```python
from build123d import *

# Parameters (mm, degrees)
SKETCH1_W           = 42
SKETCH1_H           = 22.5
BOSS_EXTRUDE1_DEPTH = 5.75
SKETCH2_W           = 10.5
SKETCH2_H           = 21.5
CUT_EXTRUDE1_DEPTH  = 4
SKETCH3_R           = 1
BOSS_EXTRUDE2_DEPTH = 8
SKETCH4_R           = 0.5
BOSS_EXTRUDE3_DEPTH = 8
SKETCH5_R           = 1.030633651
SKETCH5_W           = 20.392034512
SKETCH5_H           = 11.098868447
CUT_EXTRUDE2_DEPTH  = 0.5
SKETCH9_W           = 11.5
SKETCH9_H           = 22.5
SKETCH9_W_2         = 10.5
SKETCH9_H_2         = 21.5
CUT_EXTRUDE5_DEPTH  = 3.5
SKETCH10_W          = 11.5
SKETCH10_H          = 22.5
SKETCH10_W_2        = 10.5
SKETCH10_H_2        = 21.5
CUT_EXTRUDE6_DEPTH  = 3.5


with BuildPart() as part:
    # Sketch1 → Boss-Extrude1 (new body, symmetric)
    with BuildSketch(Plane.XY):
        Rectangle(SKETCH1_W, SKETCH1_H)
    extrude(amount=BOSS_EXTRUDE1_DEPTH, both=True)

    # Sketch2 → Cut-Extrude1 (cut)
    with BuildSketch(Plane(origin=(21, 0, 0), x_dir=(0, 0, -1), z_dir=(1, 0, 0))):
        Rectangle(SKETCH2_W, SKETCH2_H)
    cut_extrude1 = extrude(amount=-CUT_EXTRUDE1_DEPTH, mode=Mode.SUBTRACT)

    # Mirror1: Cut-Extrude1 across plane
    add(cut_extrude1.mirror(Plane(origin=(0, 0, 0), x_dir=(0, 0, 1), z_dir=(1, 0, 0))), mode=Mode.SUBTRACT)

    # Sketch3 → Boss-Extrude2 (add)
    with BuildSketch(Plane(origin=(17, 0, 0), x_dir=(0, 0, -1), z_dir=(1, 0, 0))):
        with Locations((2.259944465, 7.5)):
            Circle(SKETCH3_R)
        with Locations((2.259944465, -7.5)):
            Circle(SKETCH3_R)
    extrude(amount=BOSS_EXTRUDE2_DEPTH)

    # Sketch4 → Boss-Extrude3 (add)
    with BuildSketch(Plane.ZY.offset(17)):
        with Locations((-3.364806204, 2.988148793)):
            Circle(SKETCH4_R)
        with Locations((-3.364806204, -2.988148793)):
            Circle(SKETCH4_R)
    extrude(amount=BOSS_EXTRUDE3_DEPTH)

    # Sketch5 → Cut-Extrude2 (cut)
    with BuildSketch(Plane.XY.offset(5.75)):
        with Locations((12.976825893, 7.964601522)):
            Circle(SKETCH5_R)
        with Locations((-2.003815564, 2.9231166)):
            Rectangle(SKETCH5_W, SKETCH5_H)
    extrude(amount=-CUT_EXTRUDE2_DEPTH, mode=Mode.SUBTRACT)

    # Sketch9 → Cut-Extrude5 (cut)
    with BuildSketch(Plane(origin=(21, 0, 0), x_dir=(0, 0, -1), z_dir=(1, 0, 0))):
        Rectangle(SKETCH9_W, SKETCH9_H)
        Rectangle(SKETCH9_W_2, SKETCH9_H_2, mode=Mode.SUBTRACT)
    extrude(amount=-CUT_EXTRUDE5_DEPTH, mode=Mode.SUBTRACT)

    # Sketch10 → Cut-Extrude6 (cut)
    with BuildSketch(Plane.ZY.offset(21)):
        Rectangle(SKETCH10_W, SKETCH10_H)
        Rectangle(SKETCH10_W_2, SKETCH10_H_2, mode=Mode.SUBTRACT)
    extrude(amount=-CUT_EXTRUDE6_DEPTH, mode=Mode.SUBTRACT)


solid = part.part
```
For this review, take the finished solid that the model builds, in its own axes (mm). A direction names the side the tool comes from. Round coordinates to 2 decimals unless told otherwise and drop trailing zeros. Loops run counter-clockwise (first coordinate to the right, second up) from the corner with the lowest first, then second, coordinate; pieces in that order, holes last.
(1) We need section D-D (x = -5). Give the boundary of the cut face in (y, z).
Returned:
outline: (-11.25, -5.75) - (11.25, -5.75) - (11.25, 5.75) - (8.47, 5.75) - (8.47, 5.25) - (-2.63, 5.25) - (-2.63, 5.75) - (-11.25, 5.75) - close
(2) Mouldability with a two-part tool opening along Z and no side actions: class faces 1 (the flat face through (-2, 3, 5.25)), 2 (the flat face through (0, 11.25, 0)), 3 (the flat face through (-17, 0, 0)) as released by +Z, released by -Z, zero draft, split by the parting line, or undercut.
Returned:
face 1: released by +Z
face 2: zero draft
face 3: undercut
(3) We need section A-A (z = 4.25). Give the boundary of the cut face in (x, y), plus the area to 3 significant figures.
Returned:
outline: (-17.5, -11.25) - (17.5, -11.25) - (17.5, -10.75) - (17, -10.75) - (17, 10.75) - (17.5, 10.75) - (17.5, 11.25) - (-17.5, 11.25) - (-17.5, 10.75) - (-17, 10.75) - (-17, -10.75) - (-17.5, -10.75) - close
area: 766 mm2
(4) We need section B-B (y = -0.5). Give the boundary of the cut face in (x, z), plus the area to 3 significant figures.
Returned:
outline: (-17.5, -5.75) - (17.5, -5.75) - (17.5, -5.25) - (17, -5.25) - (17, 5.25) - (17.5, 5.25) - (17.5, 5.75) - (8.19, 5.75) - (8.19, 5.25) - (-12.2, 5.25) - (-12.2, 5.75) - (-17.5, 5.75) - (-17.5, 5.25) - (-17, 5.25) - (-17, -5.25) - (-17.5, -5.25) - close
area: 382 mm2
(5) Clearance check with flat-ended pins moving along their axes: P1, Ø1.5, axis at y = 1, z = 0.5, coming from the -X side; P2, Ø1.5, axis at x = -18.5, z = -0.5, coming from the +Y side; P3, Ø6, axis at y = 9, z = 3, coming from the -X side; P4, Ø4, axis at y = 7.5, z = 1, coming from the +X side. State where each tip first meets the part, or that it passes through.
Returned:
P1: stops at x = -17
P2: passes through
P3: stops at x = -17.5
P4: stops at x = 17
(6) We need section C-C (x = 21). Give the boundary of the cut face in (y, z), plus the area to 3 significant figures.
Returned:
outline: circle Ø2 at (-7.5, -2.26); circle Ø2 at (7.5, -2.26)
area: 6.28 mm2
(7) Wall thickness on line 1 along X through (y, z) = (3, 5.5); line 2 along X through (y, z) = (-9.75, -3.5); line 3 along Z through (x, y) = (-9.5, -2.25): over which ranges is each line inside the solid? List them lowest first.
Returned:
line 1: x = -17.5 to -12.2, 8.19 to 17.5
line 2: x = -17 to 17
line 3: z = -5.75 to 5.25
(8) Tool access review of faces 4 (the flat face through (25, 8, -2)), 5 (the cylindrical face through (20.94, -6.51, -2.13)), 6 (the flat face through (13, 8, 5.25)), 7 (the cylindrical face through (-20.944, 2.545, -3.134)): name each direction out of +Z, -Z, +X, -X, +Y, -Y from which nothing blocks a thin tool from reaching the whole face with its end or side.
Returned:
face 4: +Z, -Z, +X, +Y, -Y
face 5: +X
face 6: +Z
face 7: -X
